Autodesk Inventor part; units mm, degrees
ref_plane "YZ Plane" through (0, 0, 0) normal (1, 0, 0) x (0, 1, 0)
ref_plane "XZ Plane" through (0, 0, 0) normal (0, 1, 0) x (-1, 0, 0)
ref_plane "XY Plane" through (0, 0, 0) normal (0, 0, 1) x (1, 0, 0)
sketch "Sketch1" plane through (0, 0, 0) normal (0, 0, 1) x (1, 0, 0)
  line L0 (7.3323, 0) -> (3.6662, -6.35)
  line L1 (3.6662, -6.35) -> (-3.6662, -6.35)
  line L2 (-3.6662, -6.35) -> (-7.3323, 0)
  line L3 (-7.3323, 0) -> (-3.6662, 6.35)
  line L4 (-3.6662, 6.35) -> (3.6662, 6.35)
  line L5 (3.6662, 6.35) -> (7.3323, 0)
  circle A0 centre (0, 0) radius 9.652
  point P0 (0, 0)
  point P1 (0, 0)
  dimension "d0" = 19.304
  dimension "d1" = 12.7
extrude "Extrusion1" add sketch "Sketch1" along normal blind 6.35
properties part number "0.25 Spacer"
CAD build for the part. Positions are in the model's coordinates, mm. A direction names the side the tool comes from. Round coordinates to 2 decimals unless told otherwise and drop trailing zeros. Order: outer loops, then holes, each group sorted by start corner. A loop starts at its lowest first (then second) coordinate and runs counter-clockwise, first axis right, second up. Notation, with made-up numbers: (-36, -14) -> (-28, -14) arc R17 ccw to (-28, -10) -> close; hole circle Ø10 at (-27.75, 11.25). An arc over 180 degrees is marked (long way). Write item = value, one per line. Start each with the question number.
(1) Cut at B-B, the plane y = 3.25. List the corners of the cut face in (x, z).
(2) Pin check, flat tips, straight feed: P1, Ø1.5, axis at x = -3.5, z = 2.5, coming from the -Y side; P2, Ø3, axis at x = -7.5, z = 5.5, coming from the +Y side. Stop position of each tip, or through.
(3) Which spindle directions (+Z, -Z, +X, -X, +Y, -Y) get a long thin tool onto all of the face, cutting with end or side? Do faces 4 (the flat face through (6.3, 2.3, 0)), 5 (the flat face through (-5.525, 3.131, 3.131)). Say none if no direction does.
(4) Probe line 1 (X direction, y = -2.5, z = 2); line 2 (Y direction, x = -3.5, z = 3.5); line 3 (Y direction, x = 7, z = 1.5). List the from-to ranges inside material, lowest first. Write a range as [from, to].
(5) Cut at C-C, the plane z = 5.25. List the corners of the cut face in (x, y).
(6) Pull direction Y, two halves, no side cores. Call faces 1 (the cylindrical face through (-7.66, 5.87, 3.13)), 2 (the flat face through (0, -6.35, 3)), 3 (the flat face through (6.3, 2.3, 6.35)): released by +Y, released by -Y, zero draft, split by the parting line, or undercut.
(7) Cut at A-A, the plane x = 0. List the corners of the cut face in (y, z).
Model answer:
q1.outline = (-9.09, 0) -> (-5.46, 0) -> (-5.46, 6.35) -> (-9.09, 6.35) -> close; (5.46, 0) -> (9.09, 0) -> (9.09, 6.35) -> (5.46, 6.35) -> close
q2.P1 = -9.25
q2.P2 = 7.56
q3.face_4 = -Z, +X, -X, +Y, -Y
q3.face_5 = +Z, -Z
q4.line_1 = [-9.32, -5.89], [5.89, 9.32]
q4.line_2 = [-9, -6.35], [6.35, 9]
q4.line_3 = [-6.65, -0.58], [0.58, 6.65]
q5.outline = circle Ø19.3 at (0, 0); hole (-7.33, 0) -> (-3.67, -6.35) -> (3.67, -6.35) -> (7.33, 0) -> (3.67, 6.35) -> (-3.67, 6.35) -> close
q6.face_1 = split by the parting line
q6.face_2 = undercut
q6.face_3 = zero draft
q7.outline = (-9.65, 0) -> (-6.35, 0) -> (-6.35, 6.35) -> (-9.65, 6.35) -> close; (6.35, 0) -> (9.65, 0) -> (9.65, 6.35) -> (6.35, 6.35) -> close
